Autodesk Inventor part; units mm, degrees
ref_plane "YZ Plane" through (0, 0, 0) normal (1, 0, 0) x (0, 1, 0)
ref_plane "XZ Plane" through (0, 0, 0) normal (0, 1, 0) x (-1, 0, 0)
ref_plane "XY Plane" through (0, 0, 0) normal (0, 0, 1) x (1, 0, 0)
sketch "Sketch1" plane through (0, 0, 0) normal (0, 1, 0) x (-1, 0, 0)
  circle A0 centre (0, 0) radius 15
  circle A1 centre (0, 0) radius 4.1
  arc A2 (4.1, 0) -> (6.6908, 13.4251) centre (-45.2629, 16.4886) ccw
  line L0 (4.1, 0) -> (5.0548, -0.2974)
  line L1 (6.6908, 13.4251) -> (7.6829, 13.2996)
  arc A3 (5.0548, -0.2974) -> (7.6829, 13.2996) centre (-40.0035, 15.4643) ccw
  dimension "d0" = 30
  dimension "d1" = 8.2
  dimension "d10" = 1
  dimension "d11" = 1
extrude "Extrusion1" add sketch "Sketch1" along normal blind 2 contours A2 L0 A3 A0 | A0 A3 L0 A2
extrude "Extrusion3" add sketch "Sketch1" along normal blind 12 contours L1 A3 A0 | A0 A3 L0 A2 picked at (6.2625, 7.2317)
pattern_circular "Circular Pattern2" count 6 over 360 about axis through (0, 0, 0) along (0, 1, 0) of "Extrusion3"
equation "\"d0\" = PropDiameter"
equation "\"d1\" = PropHoleDiameter"
equation "\"d10\" = PropBladeThickness"
equation "\"d11\" = PropBladeThickness"
equation "\"d2\" = PropPlateThickness"
equation "\"d12\" = PropPlateThickness + PropDepth"
equation "\"PropHoleDiameter\" = 8.2"
equation "\"PropDepth\" = 10"
equation "\"PropPlateThickness\" = 2"
equation "\"PropBladeThickness\" = 1"
equation "\"VoluteCaseInnerSize\" = 31"
equation "\"VoluteCaseOuterSize\" = 42"
equation "\"VoluteWallThickness\" = 2"
equation "\"VoluteStartAngle\" = 25deg"
properties part number "Propeller"
Read the model definition and answer for the solid it produces. Units are mm, in the model's axes. A direction names the side the tool comes from. Coordinates: 2 decimals unless noted, no trailing zeros. Loops run counter-clockwise (first coordinate to the right, second up) from the corner with the lowest first, then second, coordinate; pieces in that order, holes last.
Q1. Consider probe 1 along Y at (x, z) = (2.5, 6.75); probe 2 along Z at (x, y) = (0, 1.5); probe 3 along X at (y, z) = (3.25, 11.5). Determine where each line is inside the solid, lowest interval first.
Q2. The part is cut by section D-D on z = -6.5. Write down the section's boundary in (x, y).
Q3. Which of the six approach directions +Z, -Z, +X, -X, +Y, -Y give full straight-line access (tool end or side, diameter ignored) to faces 5 (the face through (-8.75, 6.93, -1.71)), 6 (the face through (-3.2, 0, -3.1)), 7 (the face through (5.856, 6.93, -6.721)), 8 (the face through (9.1, 7.2, 2.7)), 9 (the face through (-13.22, 0.99, -7.09))?
Q4. The mould has two halves that part along Z. Classify faces 1 (the face through (-7.18, 5.916, 13.363)), 2 (the face through (6.1, 12, -6.6)), 3 (the face through (7.18, 5.916, -13.363)), 4 (the face through (4.571, 6.93, 0.147)): +Z half, -Z half, draft (parallel to the pull), parting line (faces both ways), or undercut.
Q5. The part is cut by section B-B on x = 0. Write down the section's boundary in (y, z), and give its area (3 significant figures).
Q6. The part is cut by section A-A on y = 5.75. Write down the section's boundary in (x, z), and give its area (3 significant figures).
Q7. The part is cut by section C-C on z = -3. Write down the section's boundary in (x, y), and give its area (3 significant figures).
Q8. Each of these flat-tipped pins is pushed along its axis until it touches: pin 1 Ø10.5 at (x, z) = (0, 0) entering from -Y; pin 2 Ø6 at (x, y) = (-2, 9) entering from +Z; pin 3 Ø6.5 at (x, z) = (-10, 4) entering from +Y; pin 4 Ø3 at (x, y) = (9, 2.5) entering from +Z. Where does it stop, or does it pass through?
Results below:
1. probe 1: y = 0 to 2
1. probe 2: z = -15 to -4.1, 4.1 to 15
1. probe 3: x = -7.57 to -6.54, 5.05 to 6.81
2. outline: (-13.52, 0) - (13.52, 0) - (13.52, 2) - (6.88, 2) - (6.88, 12) - (5.81, 12) - (5.81, 2) - (0.7, 2) - (0.7, 12) - (-0.78, 12) - (-0.78, 2) - (-13.52, 2) - close
3. face 5: +Y
3. face 6: +Z, -Z, +X, -X, -Y
3. face 7: -Z, +Y
3. face 8: +X, +Y
3. face 9: -Z, -X, +Y, -Y
4. face 1: +Z half
4. face 2: draft
4. face 3: -Z half
4. face 4: undercut
5. outline: (0, -15) - (2, -15) - (2, -7.2) - (12, -7.2) - (12, -5.74) - (2, -5.74) - (2, -4.1) - (0, -4.1) - close; (0, 4.1) - (2, 4.1) - (2, 5.74) - (12, 5.74) - (12, 7.2) - (2, 7.2) - (2, 15) - (0, 15) - close
5. area: 72.9 mm2
6. outline: (-15.36, 0) arc R47.73 ccw to (-2.27, -4.53) - (-2.05, -3.55) arc R52.05 cw to (-14.97, 0.92) - close; (-8.28, -12.51) - (-7.68, -13.3) arc R47.73 ccw to (2.78, -4.23) - (2.05, -3.55) arc R52.05 cw to start; (-7.68, 13.3) arc R47.73 ccw to (-5.05, -0.3) - (-4.1, 0) arc R52.05 cw to (-6.69, 13.43) - close; (-2.78, 4.23) - (-2.05, 3.55) arc R52.05 cw to (8.28, 12.51) - (7.68, 13.3) arc R47.73 ccw to start; (2.05, 3.55) arc R52.05 cw to (14.97, -0.92) - (15.36, 0) arc R47.73 ccw to (2.27, 4.53) - close; (4.1, 0) arc R52.05 cw to (6.69, -13.43) - (7.68, -13.3) arc R47.73 ccw to (5.05, 0.3) - close
6. area: 85.5 mm2
7. outline: (-14.7, 0) - (-2.79, 0) - (-2.79, 2) - (-4.46, 2) - (-4.46, 12) - (-8.21, 12) - (-8.21, 2) - (-14.7, 2) - close; (2.79, 0) - (14.7, 0) - (14.7, 2) - (6.08, 2) - (6.08, 12) - (5, 12) - (5, 2) - (2.79, 2) - close
7. area: 95.9 mm2
8. pin 1: stops at y = 0
8. pin 2: stops at z = 8.15
8. pin 3: stops at y = 2
8. pin 4: stops at z = 13.3
